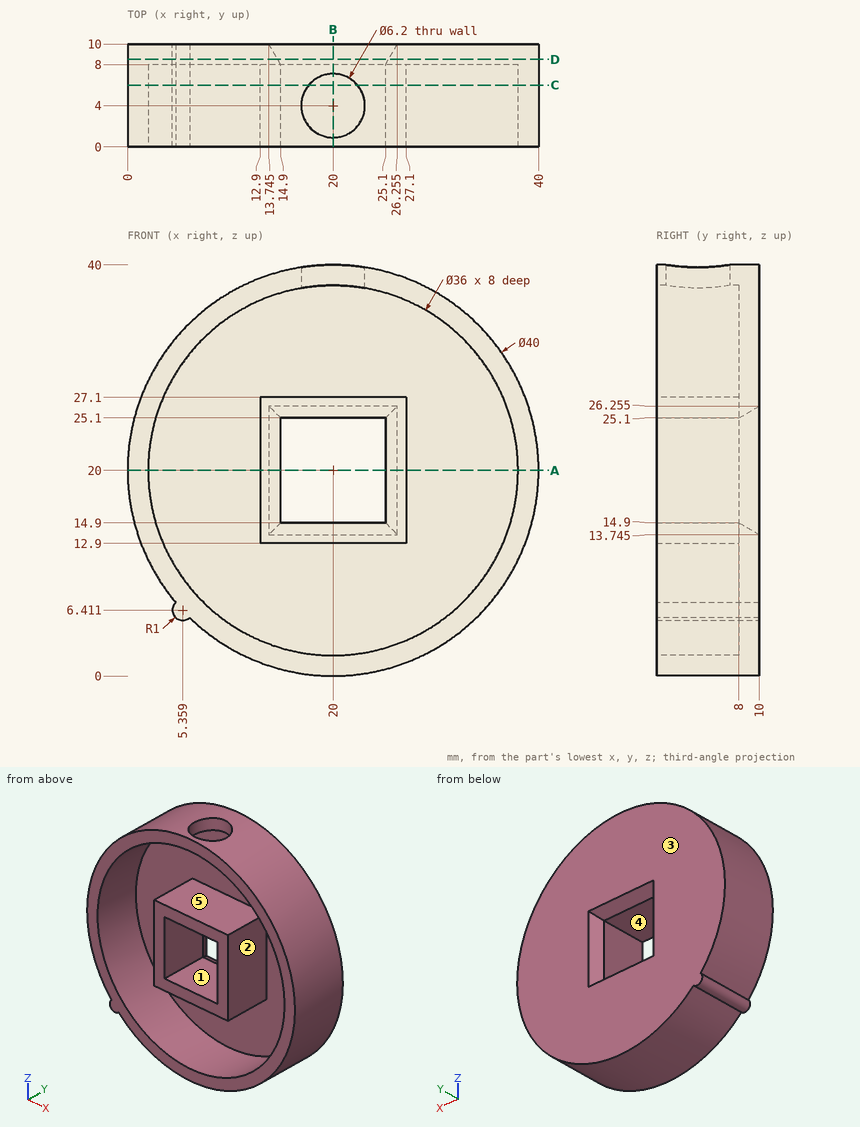
Study the drawing (mm; zero at the part's minimum x, y, z) and answer. A direction names the side the tool comes from. Round coordinates to 2 decimals unless told otherwise and drop trailing zeros. Write each loop counter-clockwise with the first axis right and the second up, starting at its lowest first coordinate (ties: lowest second). Pieces come first, ordered by that corner, then holes. Notation, with made-up numbers: (32.5, 30.25) - (81.5, 30.25) arc R11 ccw to (81.5, 37.25) - close; hole circle Ø7 at (74.5, 66). An arc over 180 degrees is marked (long way). Use CSV: the item, a comma, the result in double quotes.
Q1. Determine the mould class of the marked faces 1, 2 and 3 for opening direction Z: +Z half, -Z half, draft (parallel to the pull), parting line (faces both ways), or undercut.
Values:
face 1,"undercut"
face 2,"undercut"
face 3,"draft"
Q2. Each of these flat-tipped pins is pushed along its axis until it touches: pin 1 Ø5 at (x, y) = (6.5, 4.5) entering from -Z; pin 2 Ø1 at (x, y) = (30, 2.5) entering from +Z; pin 3 Ø2.5 at (y, z) = (3.5, 18.5) entering from -X; pin 4 Ø4 at (x, y) = (7.5, 8) entering from +Z. Where does it stop, or does it pass through?
Values:
pin 1,"stops at z = 3.3"
pin 2,"stops at z = 37.6"
pin 3,"stops at x = 0"
pin 4,"stops at z = 37.02"
Q3. Find section C-C, the plane y = 6. Write down the section's boundary in (x, z) (1 decimal).
Values:
outline,"(4.7, 7.1) arc R1 ccw to (6, 5.7) arc R20 ccw (long way) to (22.4, 39.9) - (22.4, 37.8) arc R18 cw (long way) to (17.6, 37.8) - (17.6, 39.9) arc R20 ccw to start; (12.9, 12.9) - (27.1, 12.9) - (27.1, 27.1) - (12.9, 27.1) - close; hole (14.9, 14.9) - (25.1, 14.9) - (25.1, 25.1) - (14.9, 25.1) - close"
Q4. Find section B-B, the plane x = 20. Write down the section's boundary in (y, z) (1 decimal).
Values:
outline,"(0, 0) - (10, 0) - (10, 13.7) - (8, 14.9) - (0, 14.9) - (0, 12.9) - (8, 12.9) - (8, 2) - (0, 2) - close; (0, 25.1) - (8, 25.1) - (10, 26.3) - (10, 40) - (7.1, 40) - (7.1, 38) - (8, 38) - (8, 27.1) - (0, 27.1) - close; (0, 38) - (0.9, 38) - (0.9, 40) - (0, 40) - close"
Q5. Find section D-D, the plane y = 8.5. Write down the section's boundary in (x, z) (1 decimal), then the cut area to 3 significant figures.
Values:
outline,"(4.7, 7.1) arc R1 ccw to (6, 5.7) arc R20 ccw (long way) to start; hole (14.6, 14.6) - (25.4, 14.6) - (25.4, 25.4) - (14.6, 25.4) - close"
area,"1,140 mm²"
Q6. A tool of negligible diameter and unlimited length cuts with its end or side. For the marked faces 4 and 5, from which of +Z, -Z, +X, -X, +Y, -Y can it reach the whole face along a straight path? Write none if from no direction.
Values:
face 4,"+Y, -Y"
face 5,"-Y"
Q7. Find section A-A, the plane z = 20. Write down the section's boundary in (x, y) (1 decimal), then the cut area to 3 significant figures.
Values:
outline,"(0, 0) - (2, 0) - (2, 8) - (12.9, 8) - (12.9, 0) - (14.9, 0) - (14.9, 8) - (13.7, 10) - (0, 10) - close; (25.1, 0) - (27.1, 0) - (27.1, 8) - (38, 8) - (38, 0) - (40, 0) - (40, 10) - (26.3, 10) - (25.1, 8) - close"
area,"121 mm²"
Q8. Straight lines are drawn through the part: line 1 along Z through (x, y) = (20, 2.75); line 2 along X through (y, z) = (3.25, 15.5); line 3 along Y through (x, z) = (20, 39.35). For each, find the intervals that lie inside material, in ascending order.
Values:
line 1,"z = 0 to 2, 12.9 to 14.9, 25.1 to 27.1"
line 2,"x = 0.51 to 2.57, 12.9 to 14.9, 25.1 to 27.1, 37.43 to 39.49"
line 3,"y = 0 to 0.9, 7.1 to 10"
